```python
from build123d import *

# Parameters (mm, degrees)
F0_W     = 30
F0_H     = 30
F1_DEPTH = 2.5
F2_R     = 2.8452020341
F3_DEPTH = 12.5
F4_R     = 13.1863944163
F4_R_2   = 10.5757052103
F5_DEPTH = 12.5


# Not quite as in the source:
# - a feature names something its author has since deleted; it is built from what else it names


with BuildPart() as f1:
    # F0 (on Top) → F1 (new body)
    with BuildSketch(Plane.XY):
        Rectangle(F0_W, F0_H)
    extrude(amount=F1_DEPTH)

    # F2 (on Top) → F3 (join)
    with BuildSketch(Plane.XY):
        Circle(F2_R)
    extrude(amount=F3_DEPTH)

    # F4 (on Top) → F5 (join)
    with BuildSketch(Plane.XY):
        Circle(F4_R)
        Circle(F4_R_2, mode=Mode.SUBTRACT)
    extrude(amount=F5_DEPTH)


solid = f1.part
```
For this review, take the finished solid that the model builds, in its own axes (mm). A direction names the side the tool comes from. Coordinates: 2 decimals unless noted, no trailing zeros. Write each loop counter-clockwise with the first axis right and the second up, starting at its lowest first coordinate (ties: lowest second). Pieces come first, ordered by that corner, then holes. Notation, with made-up numbers: (63.5, 14) -> (86.5, 14) arc R20 ccw to (86.5, 28) -> close; hole circle Ø7 at (31.5, 70.25). An arc over 180 degrees is marked (long way). Put each result on its own line as item: value.
Q1. Tool access review of faces 1 (the flat face through (2.2, -2.2, 2.5)), 2 (the flat face through (0, 0, 0)): name each direction out of +Z, -Z, +X, -X, +Y, -Y from which nothing blocks a thin tool from reaching the whole face with its end or side.
From the geometry:
face 1: +Z
face 2: -Z, +X, -X, +Y, -Y
Q2. Wall thickness on L1, parallel to Y at x = 0, z = 4.75; L2, parallel to Y at x = -0.75, z = 4.5: over which ranges is each line inside the solid? List them lowest first.
From the geometry:
L1: y = -13.19 to -10.58, -2.85 to 2.85, 10.58 to 13.19
L2: y = -13.17 to -10.55, -2.74 to 2.74, 10.55 to 13.17
Q3. Take a section at B-B, the plane z = 8.25. State the section outline as (x, y) points, then the cut area to 3 significant figures.
From the geometry:
outline: circle Ø26.37 at (0, 0); circle Ø5.69 at (0, 0); hole circle Ø21.15 at (0, 0)
area: 220 mm2
Q4. Take a section at D-D, the plane y = -6.5. State the section outline as (x, z) points, then the cut area to 3 significant figures.
From the geometry:
outline: (-15, 0) -> (15, 0) -> (15, 2.5) -> (11.47, 2.5) -> (11.47, 12.5) -> (8.34, 12.5) -> (8.34, 2.5) -> (-8.34, 2.5) -> (-8.34, 12.5) -> (-11.47, 12.5) -> (-11.47, 2.5) -> (-15, 2.5) -> close
area: 138 mm2
Q5. Clearance check with flat-ended pins moving along their axes: pin 1 Ø6 at (x, z) = (9.5, 5) entering from -Y; pin 2 Ø1.5 at (x, z) = (11, 8.5) entering from -Y; pin 3 Ø4 at (x, y) = (0.5, -5) entering from +Z; pin 4 Ø3 at (x, z) = (11.5, 6.5) entering from -Y. State where each tip first meets the part, or that it passes through.
From the geometry:
pin 1: stops at y = -15
pin 2: stops at y = -8.3
pin 3: stops at z = 2.5
pin 4: stops at y = -8.6
Q6. Take a section at A-A, the plane y = 0. State the section outline as (x, z) points.
From the geometry:
outline: (-15, 0) -> (15, 0) -> (15, 2.5) -> (13.19, 2.5) -> (13.19, 12.5) -> (10.58, 12.5) -> (10.58, 2.5) -> (2.85, 2.5) -> (2.85, 12.5) -> (-2.85, 12.5) -> (-2.85, 2.5) -> (-10.58, 2.5) -> (-10.58, 12.5) -> (-13.19, 12.5) -> (-13.19, 2.5) -> (-15, 2.5) -> close
Q7. The part is to be moulded in two halves that separate along X. For faces 3 (the flat face through (-15, 0, 1)), 4 (the flat face through (15, 0, 1)), 5 (the cylindrical face through (4.88, -9.382, 7.43)), say which applies: +X half, -X half, draft (parallel to the pull), parting line (faces both ways), or undercut.
From the geometry:
face 3: -X half
face 4: +X half
face 5: undercut
